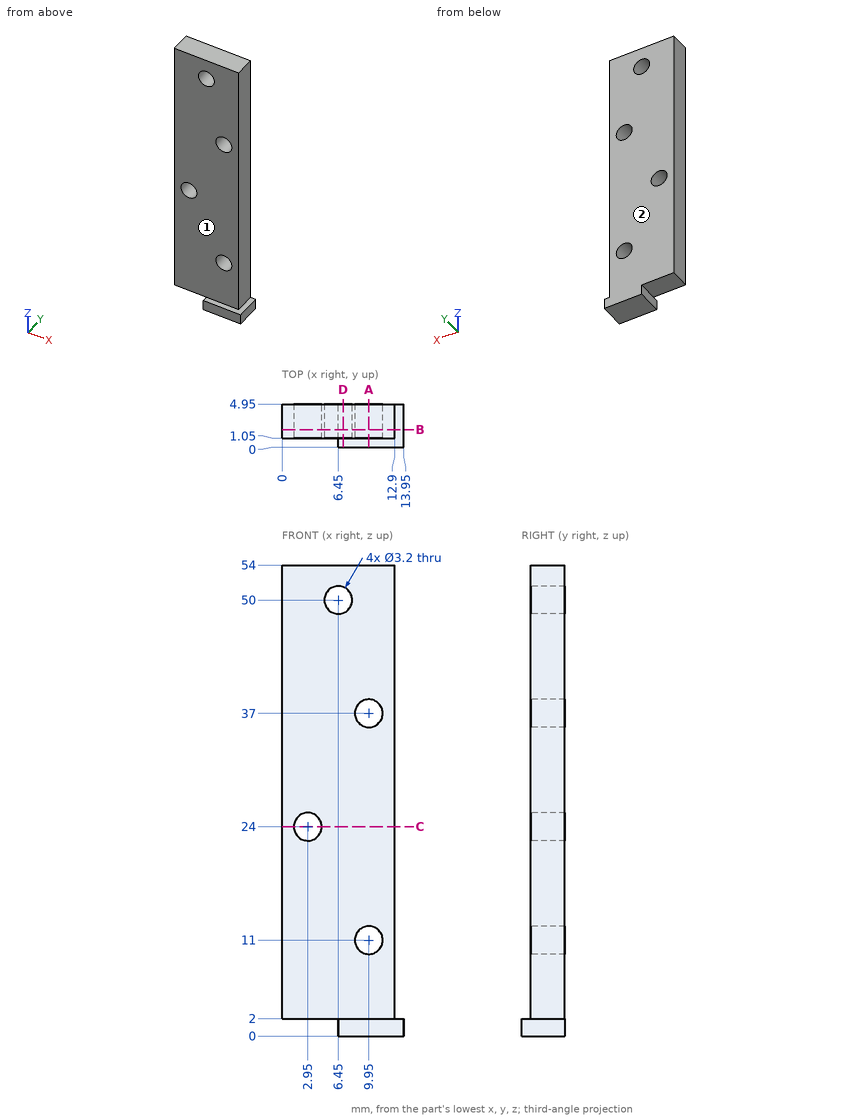
Verification items for this drawing (mm, ordinates from the low corner). A direction names the side the tool comes from. Coordinates: 2 decimals unless noted, no trailing zeros. Order: outer loops, then holes, each group sorted by start corner. A loop starts at its lowest first (then second) coordinate and runs counter-clockwise, first axis right, second up. Notation, with made-up numbers: (-7.5, -33.75) - (49.5, -33.75) arc R30 cw to (49.5, -2.75) - close; hole circle Ø11 at (-20.5, -27). An arc over 180 degrees is marked (long way). Use one line per item in the form item = value.
1. Section check B-B (y = 2). Record the boundary of the cut face in (x, z).
Here are the results:
outline = (0, 2) - (6.45, 2) - (6.45, 0) - (13.95, 0) - (13.95, 2) - (12.9, 2) - (12.9, 54) - (0, 54) - close; hole circle Ø3.2 at (2.95, 24); hole circle Ø3.2 at (6.45, 50); hole circle Ø3.2 at (9.95, 11); hole circle Ø3.2 at (9.95, 37)
2. Scan lines: line 1 (Z direction, x = 9.95, y = 2); line 2 (Z direction, x = 9.5, y = 1.7); line 3 (Z direction, x = 2.95, y = 2.2). Record each from-to range of solid material in increasing order.
Here are the results:
line_1 = 0 to 9.4, 12.6 to 35.4, 38.6 to 54
line_2 = 0 to 9.46, 12.54 to 35.46, 38.54 to 54
line_3 = 2 to 22.4, 25.6 to 54
3. Section check D-D (x = 7). Record the boundary of the cut face in (y, z), then the cut area to 3 significant figures.
Here are the results:
outline = (0, 0) - (4.95, 0) - (4.95, 48.5) - (1.05, 48.5) - (1.05, 2) - (0, 2) - close; (1.05, 51.5) - (4.95, 51.5) - (4.95, 54) - (1.05, 54) - close
area = 201 mm²
4. Section check A-A (x = 9.95). Record the boundary of the cut face in (y, z), then the cut area to 3 significant figures.
Here are the results:
outline = (0, 0) - (4.95, 0) - (4.95, 9.4) - (1.05, 9.4) - (1.05, 2) - (0, 2) - close; (1.05, 12.6) - (4.95, 12.6) - (4.95, 35.4) - (1.05, 35.4) - close; (1.05, 38.6) - (4.95, 38.6) - (4.95, 54) - (1.05, 54) - close
area = 188 mm²
5. Gauge pin test, flat ends, axial feed: pin 1 (0.6 mm diameter, centred on y = 3, z = 1.5, fed in from -X); pin 2 (6.5 mm diameter, centred on x = 7, z = 31.5, fed in from -Y); pin 3 (2 mm diameter, centred on y = 2, z = 5.5, fed in from +X); pin 4 (1.9 mm diameter, centred on x = 9.95, z = 11, fed in from -Y). Record the tip position at first contact, or that the pin passes through.
Here are the results:
pin_1 = 6.45
pin_2 = 1.05
pin_3 = 12.9
pin_4 = through
6. Section check C-C (z = 24). Record the boundary of the cut face in (x, y), then the cut area to 3 significant figures.
Here are the results:
outline = (0, 1.05) - (1.35, 1.05) - (1.35, 4.95) - (0, 4.95) - close; (4.55, 1.05) - (12.9, 1.05) - (12.9, 4.95) - (4.55, 4.95) - close
area = 37.8 mm²
7. Access from +Z, -Z, +X, -X, +Y, -Y to the whole of each face (thin tool, end or side, straight path). Record for the marked faces 1 and 2.
Here are the results:
face_1 = +Z, +X, -X, -Y
face_2 = +Z, -Z, +X, -X, +Y
